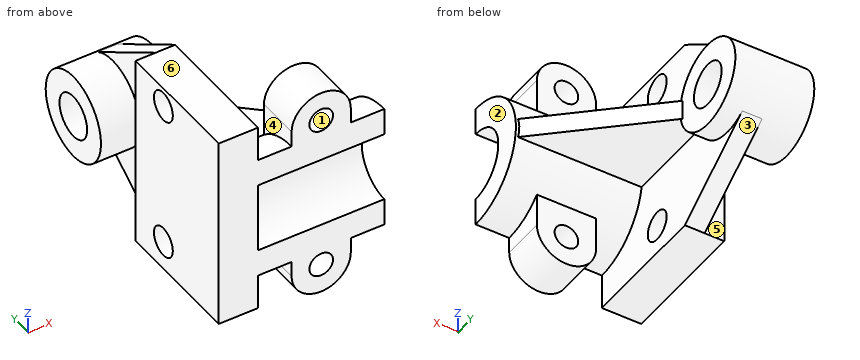
from build123d import *

# Parameters (mm, degrees)
SKETCH2_W            = 20
SKETCH2_H            = 66
BOSS_EXTRUDE1_DEPTH  = 100
SKETCH3_R            = 11
BOSS_EXTRUDE2_DEPTH  = 10
BOSS_EXTRUDE3_START  = 10
SKETCH4_R            = 22
SKETCH4_R_2          = 11
BOSS_EXTRUDE3_DEPTH  = 10
SKETCH5_R            = 22
SKETCH5_R_2          = 11
BOSS_EXTRUDE4_DEPTH  = 40
BOSS_EXTRUDE5_DEPTH  = 64
BOSS_EXTRUDE10_DEPTH = 5
SKETCH16_R           = 6
BOSS_EXTRUDE11_DEPTH = 22
SKETCH18_R           = 7.5
CUT_EXTRUDE2_DEPTH   = 22


with BuildPart() as part:
    # Sketch2 → Boss-Extrude1 (new body)
    with BuildSketch(Plane.XY):
        with Locations((-12.101382488, 33)):
            Rectangle(SKETCH2_W, SKETCH2_H)
    extrude(amount=-BOSS_EXTRUDE1_DEPTH)

    # Sketch3 → Boss-Extrude2 (add)
    # profile 1 of 2: a face of its own
    with BuildSketch(Plane(origin=(-2.101382488, 0, 0), x_dir=(0, 0, -1), z_dir=(1, 0, 0))):
        with BuildLine():
            Line((31.462791547, 111.847864903), (0, 66))
            Line((0, 66), (100, 66))
            Line((100, 66), (68.537208453, 111.847864903))
            ThreePointArc((68.537208453, 111.847864903), (71.116564422, 106.171766928), (72, 100))
            ThreePointArc((72, 100), (43.828233072, 78.883435578), (31.462791547, 111.847864903))
        make_face()
    # profile 2 of 2: a face of its own
    with BuildSketch(Plane(origin=(-2.101382488, 0, 0), x_dir=(0, 0, -1), z_dir=(1, 0, 0))):
        with BuildLine():
            Line((32.277524622, 113.035101322), (31.462791547, 111.847864903))
            ThreePointArc((31.462791547, 111.847864903), (43.828233072, 78.883435578), (72, 100))
            ThreePointArc((72, 100), (71.116564422, 106.171766928), (68.537208453, 111.847864903))
            Line((68.537208453, 111.847864903), (67.722475378, 113.035101322))
            ThreePointArc((67.722475378, 113.035101322), (50, 122), (32.277524622, 113.035101322))
        make_face()
        with Locations(Location((50, 100, 0), (0, 0, 90))):
            Circle(SKETCH3_R, mode=Mode.SUBTRACT)
    extrude(amount=-BOSS_EXTRUDE2_DEPTH)

    # Sketch4 → Boss-Extrude3 (add)
    with BuildSketch(Plane(origin=(-2.101382488, 0, 0), x_dir=(0, 0, -1), z_dir=(1, 0, 0)).offset(BOSS_EXTRUDE3_START)):
        with Locations(Location((50, 100, 0), (0, 0, 90))):
            Circle(SKETCH4_R)
        with Locations(Location((50, 100, 0), (0, 0, 90))):
            Circle(SKETCH4_R_2, mode=Mode.SUBTRACT)
    extrude(amount=-BOSS_EXTRUDE3_DEPTH)

    # Sketch5 → Boss-Extrude4 (add)
    with BuildSketch(Plane(origin=(7.898617512, 0, 0), x_dir=(0, 0, -1), z_dir=(1, 0, 0))):
        with Locations(Location((50, 100, 0), (0, 0, 90))):
            Circle(SKETCH5_R)
        with Locations(Location((50, 100, 0), (0, 0, 90))):
            Circle(SKETCH5_R_2, mode=Mode.SUBTRACT)
    extrude(amount=-BOSS_EXTRUDE4_DEPTH)

    # Sketch6 → Boss-Extrude5 (add)
    with BuildSketch(Plane(origin=(-2.101382488, 0, 0), x_dir=(0, 0, -1), z_dir=(1, 0, 0))):
        with BuildLine():
            ThreePointArc((32, 0), (50, 18), (68, 0))
            Line((68, 0), (82, 0))
            ThreePointArc((82, 0), (50, 32), (18, 0))
            Line((18, 0), (32, 0))
        make_face()
    extrude(amount=BOSS_EXTRUDE5_DEPTH)

    # Sketch9 → Boss-Extrude10 (add, symmetric)
    with BuildSketch(Plane(origin=(0, 0, -50), x_dir=(-1, 0, 0), z_dir=(0, 0, -1))):
        Polygon((-61.898617512, 30.402989501), (4.356494358, 30.402989501), (4.356494358, 79.707135775), (-7.898617512, 79.707135775), align=None)
    extrude(amount=BOSS_EXTRUDE10_DEPTH, both=True)

    # Sketch16 → Boss-Extrude11 (add)
    # profile 1 of 2: a face of its own
    with BuildSketch(Plane.XZ):
        with BuildLine():
            Line((14.898617512, -32), (14.898617512, -10))
            ThreePointArc((14.898617512, -10), (29.898617512, 5), (44.898617512, -10))
            Line((44.898617512, -10), (44.898617512, -32))
            Line((44.898617512, -32), (14.898617512, -32))
        make_face()
        with Locations((29.898617512, -10)):
            Circle(SKETCH16_R, mode=Mode.SUBTRACT)
    # profile 2 of 2: a face of its own
    with BuildSketch(Plane.XZ):
        with BuildLine():
            Line((14.898617512, -68), (14.898617512, -90))
            ThreePointArc((14.898617512, -90), (29.898617512, -105), (44.898617512, -90))
            Line((44.898617512, -90), (44.898617512, -68))
            Line((44.898617512, -68), (14.898617512, -68))
        make_face()
        with Locations((29.898617512, -90)):
            Circle(SKETCH16_R, mode=Mode.SUBTRACT)
    extrude(amount=-BOSS_EXTRUDE11_DEPTH)

    # Sketch18 → Cut-Extrude2 (cut)
    with BuildSketch(Plane(origin=(-2.101382488, 0, 0), x_dir=(0, 0, -1), z_dir=(1, 0, 0))):
        with Locations(Location((10, 44, 0), (0, 0, 90))):
            Circle(SKETCH18_R)
        with Locations(Location((85, 44, 0), (0, 0, 90))):
            Circle(SKETCH18_R)
    extrude(amount=-CUT_EXTRUDE2_DEPTH, mode=Mode.SUBTRACT)


solid = part.part
CAD build for the part. Positions are in the model's coordinates, mm. Face numbers are marked on the shaded views. A direction names the side the tool comes from. Round coordinates to 2 decimals unless told otherwise and drop trailing zeros. Write each loop counter-clockwise with the first axis right and the second up, starting at its lowest first coordinate (ties: lowest second). Pieces come first, ordered by that corner, then holes. Notation, with made-up numbers: M 29,75 L 40,75 A30 ccw 40,109 Z; hole C 22,-33 d7. An arc over 180 degrees is marked long. Put each result on its own line as item: value. Start each with the question number.
1) Saw through at C-C, the plane z = -75.5. Write the cut outline in (x, y).
2) Drill centre lines: probe 1 along Z at (x, y) = (-15, 44); probe 2 along Z at (x, y) = (-2, 100); probe 3 along X at (y, z) = (9.5, -6.5). Where is each one in solid material? Low to high. Write a range as [from, to].
3) Pin check, flat tips, straight feed: pin 1 Ø9 at (y, z) = (44, -85) entering from -X (3 decimals); pin 2 Ø24 at (y, z) = (44, -10) entering from +X; pin 3 Ø13.5 at (y, z) = (14.5, -18) entering from -X; pin 4 Ø4 at (y, z) = (18, -94) entering from +X. Stop position of each tip, or through.
4) Pull direction Z, two halves, no side cores. Call the marked faces 1, 2 and 3: pulls with the +Z half, pulls with the -Z half, needs draft (parallel to the pull), parting line crosses it, or undercut.
5) 3-axis set-ups, long thin cutter, end or side, ignore diameter. For the marked faces 4, 5 and 6: which of +Z, -Z, +X, -X, +Y, -Y reach the whole face in a straight line?
6) Saw through at B-B, the plane x = -5. Write the cut outline in (y, z).
7) Saw through at A-A, the plane y = 100. Write the cut outline in (x, z).
8) Saw through at D-D, the plane x = 43. Write the cut outline in (y, z), and give its area (3 significant figures).
Resolved:
1. outline: M -22.1,0 L 61.9,0 L 61.9,19.33 L 44.9,19.33 L 44.9,22 L 14.9,22 L 14.9,19.33 L -2.1,19.33 L -2.1,101.7 L -12.1,101.7 L -12.1,66 L -22.1,66 Z
2. probe 1: [-100, -92.5], [-77.5, -17.5], [-2.5, 0]
2. probe 2: [-72, -61], [-39, -28]
2. probe 3: [-22.1, -2.1], [15.31, 25.03], [34.77, 44.48]
3. pin 1: through
3. pin 2: x = -2.1
3. pin 3: x = -22.1
3. pin 4: x = 44.76
4. face 1: undercut
4. face 2: needs draft
4. face 3: pulls with the -Z half
5. face 4: +Z, +Y
5. face 5: +Z, -Z, -X
5. face 6: +Z, -X, +Y, -Y
6. outline: M 0,-100 L 66,-100 L 111.85,-68.54 A22 ccw 111.85,-31.46 L 66,0 L 0,0 Z; hole C 44,-85 d15; hole C 44,-10 d15; hole C 100,-50 d22
7. outline: M -32.1,-72 L -12.1,-72 L -12.1,-76.67 L -2.1,-76.67 L -2.1,-72 L 7.9,-72 L 7.9,-61 L -32.1,-61 Z; M -32.1,-39 L 7.9,-39 L 7.9,-28 L -2.1,-28 L -2.1,-23.33 L -12.1,-23.33 L -12.1,-28 L -32.1,-28 Z
8. outline: M 0,-97.3 L 22,-97.3 L 22,-73.24 A32 ccw 31.61,-55 L 47.66,-55 L 47.66,-45 L 31.61,-45 A32 ccw 22,-26.76 L 22,-2.7 L 0,-2.7 L 0,-32 A18 cw 0,-68 Z
8. area: 2,050 mm²
